Here's how the part is built. I have some questions about the finished solid (model axes, mm). A direction names the side the tool comes from. Give positions to 0.01 mm unless a question says otherwise; leave off trailing zeros. Order: outer loops, then holes, each group sorted by start corner. A loop starts at its lowest first (then second) coordinate and runs counter-clockwise, first axis right, second up. Notation, with made-up numbers: (65, 77.25) -> (116, 77.25) arc R6 cw to (116, 83.25) -> close; hole circle Ø6 at (-25, -29). An arc over 180 degrees is marked (long way). Write each question's results on one line, items separated by ' | '. Start each with the question number.
Q1. Imagine slicing it at B-B, the plane x = 0. Please give me the cut outline in (y, z), then the cut area to 3 significant figures.
Q2. For faces 4 (the face through (0, 288.404, 49)), 5 (the face through (1, 281.104, 52)), 6 (the face through (11.33, 279.59, 47.13)), which set-ups out of +Z, -Z, +X, -X, +Y, -Y let a thin tool reach every point of the face, with its end or its side?
Q3. Imagine slicing it at A-A, the plane y = 339.5. Please give me the cut outline in (x, z), then the cut area to 3 significant figures.
Q4. Thinking about a two-plate mould opening in Y: for faces 1 (the face through (0.41, 279.73, 51.96)), 2 (the face through (3.3, 284, 50)), 3 (the face through (-2.3, 278.404, 50)), which applies, pulls with the +Y half, pulls with the -Y half, needs draft (parallel to the pull), parting line crosses it, or undercut?
Q5. I'm going to push flat-ended pins straight in: pin 1 (10 mm diameter, centred on x = 5, y = 332.5, fed in from +Z); pin 2 (7.5 mm diameter, centred on x = 1, z = 51.5, fed in from +Y); pin 3 (3.5 mm diameter, centred on x = -17.5, y = 337.5, fed in from +Z); pin 4 (7.5 mm diameter, centred on y = 285.5, z = 51, fed in from -X). Where does each tip first touch, or does it pass through?
Q6. Imagine slicing it at D-D, the plane y = 284. Please give me the cut outline in (x, z), then the cut area to 3 significant figures.
Q7. I need wall thicknesses on line 1 along X through (y, z) = (318.5, 44.75); line 2 along Z through (x, y) = (0, 279.4); line 3 along Y through (x, z) = (-0.5, 45). Which ranges of each line are inside material? Lowest first, please. Write a range as [from, to].
Q8. Imagine slicing it at C-C, the plane z = 45.25. Please give me the cut outline in (x, y), then the cut area to 3 significant figures.
```python
from build123d import *

# Parameters (mm, degrees)
SALIENTE_EXTRUIR1_DEPTH             = 3
CROQUIS2_W                          = 10
CROQUIS2_H                          = 10
SALIENTE_EXTRUIR2_DEPTH             = 10
CROQUIS3_W                          = 6.2
CROQUIS3_H                          = 6.2
CORTAR_EXTRUIR1_DEPTH               = 349.280563017
NGULO_START                         = 278.403728499
NGULO_DE_SALIDA1_DEPTH              = 10
NGULO_START_2                       = 46.606431878
NGULO_DE_SALIDA1_2_DEPTH            = 11.393568122
DI_METRO_DE_TALADRO_3_8_3_8_1_D     = 3.8
DI_METRO_DE_TALADRO_3_8_3_8_1_DEPTH = 2.9
REDONDEO1_R                         = 0.4
CROQUIS7_W                          = 7
CROQUIS7_H                          = 10
SALIENTE_EXTRUIR3_DEPTH             = 3
CROQUIS8_W                          = 6.6
CROQUIS8_H                          = 6.6
CORTAR_EXTRUIR2_DEPTH               = 359.256088776


with BuildPart() as part:
    # Croquis1 → Saliente-Extruir1 (new body)
    with BuildSketch(Plane(origin=(0, 0, 43.606431878), x_dir=(-1, 0, 0), z_dir=(0, 0, -1))):
        with BuildLine():
            Line((-21, 338.403728499), (-21, 281.403728499))
            Line((-21, 281.403728499), (-5, 278.403728499))
            Line((-5, 278.403728499), (5, 278.403728499))
            Line((5, 278.403728499), (21, 281.403728499))
            Line((21, 281.403728499), (21, 338.403728499))
            ThreePointArc((21, 338.403728499), (20.094205089, 343.232030478), (17.5, 347.403728499))
            ThreePointArc((17.5, 347.403728499), (14.905794911, 343.232030478), (14, 338.403728499))
            Line((14, 338.403728499), (14, 288.403728499))
            Line((14, 288.403728499), (-14, 288.403728499))
            Line((-14, 288.403728499), (-14, 338.403728499))
            ThreePointArc((-14, 338.403728499), (-14.905794911, 343.232030478), (-17.5, 347.403728499))
            ThreePointArc((-17.5, 347.403728499), (-20.094205089, 343.232030478), (-21, 338.403728499))
        make_face()
    extrude(amount=-SALIENTE_EXTRUIR1_DEPTH)

    # Croquis2 → Saliente-Extruir2 (add)
    with BuildSketch(Plane.XY.offset(46.606431878)):
        with Locations((0, 283.403728499)):
            Rectangle(CROQUIS2_W, CROQUIS2_H)
    extrude(amount=SALIENTE_EXTRUIR2_DEPTH)

    # Croquis3 → Cortar-Extruir1 (cut, through all)
    with BuildSketch(Plane.XY.offset(56.606431878)):
        with Locations((0, 284.403728499)):
            Rectangle(CROQUIS3_W, CROQUIS3_H)
    extrude(amount=-CORTAR_EXTRUIR1_DEPTH, mode=Mode.SUBTRACT)

    # Ángulo de salida1: read off the stored shape, not the designer's step
    # Ángulo de salida1 outline → Ángulo de salida1 (add)
    with BuildSketch(Plane(origin=(0, 0, 0), x_dir=(1, 0, 0), z_dir=(0, 1, 0)).offset(NGULO_START)):
        Polygon((-5, -46.606431878), (-14, -46.606431878), (-5, -56.606431878), align=None)
        Polygon((5, -46.606431878), (5, -56.606431878), (14, -46.606431878), align=None)
    extrude(amount=NGULO_DE_SALIDA1_DEPTH)

    # ngulo de salida1 2 outline → ngulo de salida1 2 (cut)
    with BuildSketch(Plane.XY.offset(NGULO_START_2)):
        Polygon((-5, 278.403728499), (-16, 280.466228499), (-16, 278.403728499), align=None)
        Polygon((15, 280.278728499), (5, 278.403728499), (15, 278.403728499), align=None)
    extrude(amount=NGULO_DE_SALIDA1_2_DEPTH, mode=Mode.SUBTRACT)

    # Diámetro de taladro Ø3.8 (3.8)1
    with Locations(Plane(origin=(0, 281.303728499, 0), x_dir=(1, 0, 0), z_dir=(0, 1, 0))):
        with Locations((0, -50.106431878)):
            Hole(DI_METRO_DE_TALADRO_3_8_3_8_1_D / 2, depth=DI_METRO_DE_TALADRO_3_8_3_8_1_DEPTH)

    # Redondeo1
    redondeo1_edges = [part.edges().sort_by_distance(p)[0] for p in [
        (-17.5, 347.403728499, 45.106431878),
        (17.5, 347.403728499, 45.106431878),
    ]]
    fillet(redondeo1_edges, radius=REDONDEO1_R)

    # Croquis7 → Saliente-Extruir3 (add, through all)
    with BuildSketch(Plane.XY.offset(46.606431878)):
        with BuildLine():
            Line((-14, 338.403728499), (-14, 348.403728499))
            Line((-14, 348.403728499), (-21, 348.403728499))
            Line((-21, 348.403728499), (-21, 338.403728499))
            ThreePointArc((-21, 338.403728499), (-20.175493128, 343.017556325), (-17.804035379, 347.060254302))
            ThreePointArc((-17.804035379, 347.060254302), (-17.5, 347.20032645), (-17.195964621, 347.060254302))
            ThreePointArc((-17.195964621, 347.060254302), (-14.824506872, 343.017556325), (-14, 338.403728499))
        make_face()
        with BuildLine():
            ThreePointArc((-14, 348.403728499), (-14.905794911, 353.232030478), (-17.5, 357.403728499))
            ThreePointArc((-17.5, 357.403728499), (-20.094205089, 353.232030478), (-21, 348.403728499))
            Line((-21, 348.403728499), (-14, 348.403728499))
        make_face()
        with BuildLine():
            ThreePointArc((14, 348.403728499), (14.905794911, 353.232030478), (17.5, 357.403728499))
            ThreePointArc((17.5, 357.403728499), (20.094205089, 353.232030478), (21, 348.403728499))
            Line((21, 348.403728499), (14, 348.403728499))
        make_face()
        with Locations((17.5, 343.403728499)):
            Rectangle(CROQUIS7_W, CROQUIS7_H)
    extrude(amount=-SALIENTE_EXTRUIR3_DEPTH)

    # Croquis8 → Cortar-Extruir2 (cut, through all)
    with BuildSketch(Plane.XY.offset(56.606431878)):
        with Locations((0, 284.403728499)):
            Rectangle(CROQUIS8_W, CROQUIS8_H)
    extrude(amount=-CORTAR_EXTRUIR2_DEPTH, mode=Mode.SUBTRACT)


solid = part.part
```
Geometry check:
1) outline: (278.4, 43.61) -> (281.1, 43.61) -> (281.1, 48.21) -> (278.4, 48.21) -> close; (278.4, 52.01) -> (281.1, 52.01) -> (281.1, 56.61) -> (278.4, 56.61) -> close; (287.7, 43.61) -> (288.4, 43.61) -> (288.4, 56.61) -> (287.7, 56.61) -> close | area: 33.9 mm²
2) face 4: +Z, -Z, +Y | face 5: +Z, -Z | face 6: +Z, -Z, +X, -Y
3) outline: (-21, 43.61) -> (-14, 43.61) -> (-14, 46.61) -> (-21, 46.61) -> close; (14, 43.61) -> (21, 43.61) -> (21, 46.61) -> (14, 46.61) -> close | area: 42.0 mm²
4) face 1: needs draft | face 2: undercut | face 3: pulls with the -Y half
5) pin 1: through | pin 2: y = 288.4 | pin 3: z = 46.61 | pin 4: x = -13.42
6) outline: (-21, 43.61) -> (-3.3, 43.61) -> (-3.3, 56.61) -> (-5, 56.61) -> (-14, 46.61) -> (-21, 46.61) -> close; (3.3, 43.61) -> (21, 43.61) -> (21, 46.61) -> (14, 46.61) -> (5, 56.61) -> (3.3, 56.61) -> close | area: 230 mm²
7) line 1: [-21, -14], [14, 21] | line 2: [43.61, 48.21], [52.01, 56.61] | line 3: [278.4, 281.1], [287.7, 288.4]
8) outline: (-21, 281.4) -> (-5, 278.4) -> (5, 278.4) -> (21, 281.4) -> (21, 348.4) arc R13.32 ccw to (17.5, 357.4) arc R13.32 ccw to (14, 348.4) -> (14, 288.4) -> (-14, 288.4) -> (-14, 348.4) arc R13.32 ccw to (-17.5, 357.4) arc R13.32 ccw to (-21, 348.4) -> close; hole (-3.3, 281.1) -> (3.3, 281.1) -> (3.3, 287.7) -> (-3.3, 287.7) -> close | area: 1,250 mm²
